For this review, use the dimensioned drawing (mm, ordinates from the lowest corner) and the shaded views. Coordinates: 2 decimals unless noted, no trailing zeros. Order: outer loops, then holes, each group sorted by start corner. A loop starts at its lowest first (then second) coordinate and runs counter-clockwise, first axis right, second up. Notation, with made-up numbers: M 37,-28.5 L 78,-28.5 A12 cw 78,-18.5 Z; hole C -20,-39 d9. An arc over 180 degrees is marked long. Use one line per item in the form item = value. Start each with the question number.
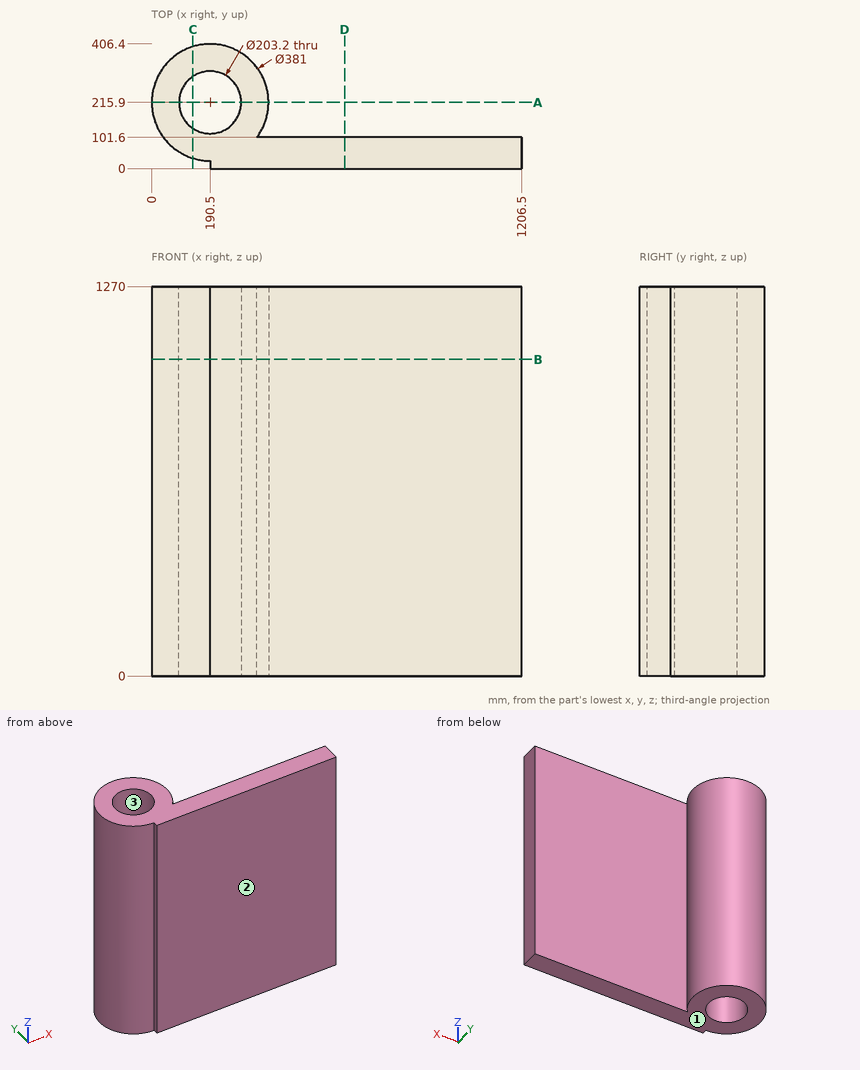
1. To check wall thickness, follow line 1 (X direction, y = 215, z = 380); line 2 (Y direction, x = 595.5, z = 385); line 3 (Y direction, x = 190, z = 881). State the ranges of each line that lie inside material, in increasing order.
2. Consider section D-D, the plane x = 629.5. Write out the cut boundary in (y, z), plus the area to 3 significant figures.
3. The part is to be moulded in two halves that separate along Y. For the marked faces 1, 2 and 3, say which applies: pulls with the +Y half, pulls with the -Y half, needs draft (parallel to the pull), parting line crosses it, or undercut.
4. Consider section C-C, the plane x = 134.5. Write out the cut boundary in (y, z), plus the area to 3 significant figures.
5. For pin 1 Ø8 at (y, z) = (239, 565.5) entering from +X; pin 2 Ø12 at (x, z) = (464.5, 198) entering from +Y; pin 3 Ø3 at (y, z) = (318.5, 263.5) entering from -X, all flat-tipped, find the tip position at first contact; note any pin that passes through.
6. Consider section A-A, the plane y = 215.9. Write out the cut boundary in (x, z).
7. Consider section B-B, the plane z = 1033. Write out the cut boundary in (x, y), plus the area to 3 significant figures.
Answers follow:
q1.line_1 = 0 to 88.9, 292.1 to 381
q1.line_2 = 0 to 101.6
q1.line_3 = 25.4 to 114.3, 317.5 to 406.4
q2.outline = M 0,0 L 101.6,0 L 101.6,1270 L 0,1270 Z
q2.area = 129,000 mm²
q3.face_1 = needs draft
q3.face_2 = pulls with the -Y half
q3.face_3 = undercut
q4.outline = M 33.82,0 L 131.13,0 L 131.13,1270 L 33.82,1270 Z; M 300.67,0 L 397.98,0 L 397.98,1270 L 300.67,1270 Z
q4.area = 247,000 mm²
q5.pin_1 = 380.04
q5.pin_2 = 101.6
q5.pin_3 = 29.04
q6.outline = M 0,0 L 88.9,0 L 88.9,1270 L 0,1270 Z; M 292.1,0 L 381,0 L 381,1270 L 292.1,1270 Z
q7.outline = M 190.5,0 L 1206.5,0 L 1206.5,101.6 L 342.9,101.6 A190.5 ccw long 190.5,25.4 Z; hole C 190.5,215.9 d203.2
q7.area = 177,000 mm²
